Print and shaded views of the part. All mm, measured from the part's lowest x, y and z. A direction names the side the tool comes from. Give positions to 0.01 mm unless a question says otherwise; leave off trailing zeros. Order: outer loops, then holes, each group sorted by start corner. A loop starts at its lowest first (then second) coordinate and runs counter-clockwise, first axis right, second up. Notation, with made-up numbers: (26.5, -18) - (53.5, -18) arc R17 cw to (53.5, -13) - close; hole circle Ø1 at (-34, 24.5). An arc over 180 degrees is marked (long way). Answer in a Markdown table with one row per item.
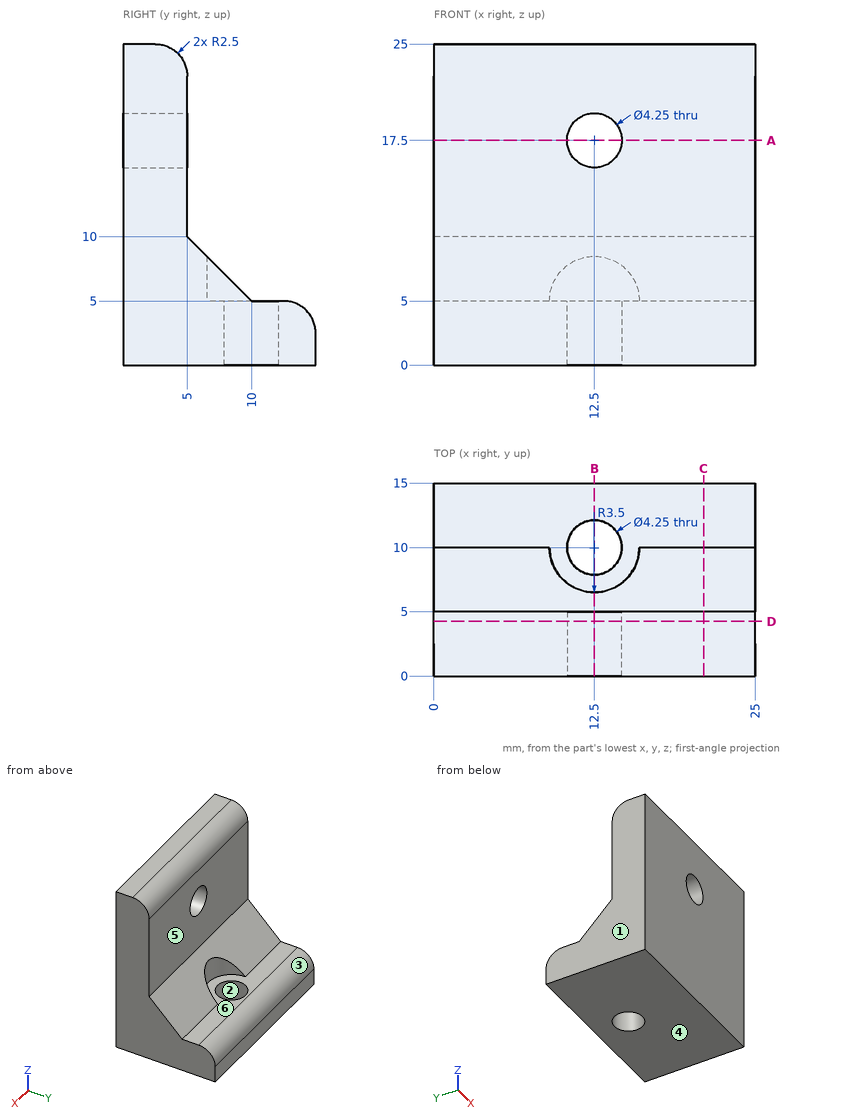
1. Two-plate mould, pull along Y, no slides. Class the marked faces 1, 2 and 3: +Y half, -Y half, draft (parallel to the pull), parting line (faces both ways), or undercut.
Check result:
| item | result |
|---|---|
| face 1 | draft |
| face 2 | undercut |
| face 3 | +Y half |
2. Cut at B-B on x = 12.5. Write the cut outline in (y, z) (3 decimals).
Check result:
| item | result |
|---|---|
| outline | (0, 0) - (7.875, 0) - (7.875, 5) - (6.5, 5) - (6.5, 8.5) - (5, 10) - (5, 15.375) - (0, 15.375) - close; (0, 19.625) - (5, 19.625) - (5, 22.5) arc R2.5 ccw to (2.5, 25) - (0, 25) - close; (12.125, 0) - (15, 0) - (15, 2.5) arc R2.5 ccw to (12.5, 5) - (12.125, 5) - close |
3. Probe line 1 (Y direction, x = 12.5, z = 1.3) (3 decimals); line 2 (X direction, y = 10, z = 3.15) (3 decimals); line 3 (Z direction, x = 13.25, y = 6.75). List the from-to ranges inside material, lowest first.
Check result:
| item | result |
|---|---|
| line 1 | y = 0 to 7.875, 12.125 to 15 |
| line 2 | x = 0 to 10.375, 14.625 to 25 |
| line 3 | z = 0 to 5 |
4. Cut at D-D on y = 4.25. Write the cut outline in (x, z) (3 decimals), and give its area (3 significant figures).
Check result:
| item | result |
|---|---|
| outline | (0, 0) - (25, 0) - (25, 24.285) - (0, 24.285) - close; hole circle Ø4.25 at (12.5, 17.5) |
| area | 593 mm² |
5. Which spindle directions (+Z, -Z, +X, -X, +Y, -Y) get a long thin tool onto all of the face, cutting with end or side? Do the marked faces 4, 5 and 6. Say none if no direction does.
Check result:
| item | result |
|---|---|
| face 4 | -Z, +X, -X, +Y, -Y |
| face 5 | +Z, +X, -X, +Y |
| face 6 | +Z, +Y |
6. Cut at C-C on x = 21. Write the cut outline in (y, z).
Check result:
| item | result |
|---|---|
| outline | (0, 0) - (15, 0) - (15, 2.5) arc R2.5 ccw to (12.5, 5) - (10, 5) - (5, 10) - (5, 22.5) arc R2.5 ccw to (2.5, 25) - (0, 25) - close |
7. Drop flat-ended pins along their axis: P1, Ø12, axis at x = 19.5, z = 6, coming from the +Y side; P2, Ø4, axis at x = 15.5, z = 18, coming from the +Y side; P3, Ø5, axis at x = 13.5, y = 8.5, coming from the +Z side; P4, Ø6, axis at x = 14.5, z = 9.5, coming from the +Y side. Give the stop position or say it passes through.
Check result:
| item | result |
|---|---|
| P1 | stops at y = 15 |
| P2 | stops at y = 5 |
| P3 | stops at z = 9 |
| P4 | stops at y = 8.31 |
8. Cut at A-A on z = 17.5. Write the cut outline in (x, y) (3 decimals).
Check result:
| item | result |
|---|---|
| outline | (0, 0) - (10.375, 0) - (10.375, 5) - (0, 5) - close; (14.625, 0) - (25, 0) - (25, 5) - (14.625, 5) - close |
